```python
from build123d import *

# Parameters (mm, degrees)
SKETCH1_W                                    = 110
SKETCH1_H                                    = 30
EXTRUDE1_DEPTH                               = 2
CUT_EXTRUDE1_DEPTH                           = 3
CHAMFER1_SIZE                                = 9
CHAMFER1_SIZE2                               = 1.5
CSK_FOR_M3_COUNTERSUNK_RAISED_HEAD_S_2_COUNT = 2
CSK_FOR_M3_COUNTERSUNK_RAISED_HEAD_S_2_PITCH = 95
CSK_FOR_M3_COUNTERSUNK_RAISED_HEAD_S_3_COUNT = 2
CSK_FOR_M3_COUNTERSUNK_RAISED_HEAD_S_3_PITCH = 97.082439195
CSK_FOR_M3_COUNTERSUNK_RAISED_HEAD_S_4_COUNT = 2
CSK_FOR_M3_COUNTERSUNK_RAISED_HEAD_S_4_PITCH = 20
M3_TAPPED_HOLE1_D                            = 3


with BuildPart() as part:
    # Sketch1 → Extrude1 (new body)
    with BuildSketch(Plane(origin=(0, 0, 0), x_dir=(1, 0, 0), z_dir=(0, 1, 0))):
        Rectangle(SKETCH1_W, SKETCH1_H)
    extrude(amount=EXTRUDE1_DEPTH)

    # Sketch2 → Cut-Extrude1 (cut, through all)
    with BuildSketch(Plane(origin=(0, 2, 0), x_dir=(-1, 0, 0), z_dir=(0, 1, 0))):
        with BuildLine():
            Line((5, 0), (5, -15))
            Line((5, -15), (-5, -15))
            Line((-5, -15), (-5, 0))
            ThreePointArc((-5, 0), (0, 5), (5, 0))
        make_face()
    extrude(amount=-CUT_EXTRUDE1_DEPTH, mode=Mode.SUBTRACT)

    # Chamfer1
    chamfer1_edges = [part.edges().sort_by_distance(p)[0] for p in [
        (0, 2, 5),
        (5, 2, -7.5),
        (-5, 2, -7.5),
    ]]
    chamfer1_side = [part.faces().sort_by_distance(p)[0] for p in [
        (-53.859824575, 2, 0),
    ]]
    chamfer(chamfer1_edges, length=CHAMFER1_SIZE, length2=CHAMFER1_SIZE2, reference=chamfer1_side[0])

    # Sketch8 → CSK for M3 Countersunk Raised Head Screw1 (revolve, cut)
    with BuildSketch(Plane(origin=(47.5, 0, -10), x_dir=(0, 0, -1), z_dir=(1, 0, 0))):
        Polygon((0, 0), (0, 2), (1.7, 2), (1.7, 1.45), (3.15, 0), align=None)
    csk_for_m3_countersunk_raised_head_screw = revolve(axis=Axis((47.5, -6.35, -10), (0, 1, 0)), mode=Mode.SUBTRACT)

    # CSK for M3 Countersunk Raised Head S 2: CSK for M3 Countersunk Raised Head Screw1 ×2
    with Locations(*[(-i * CSK_FOR_M3_COUNTERSUNK_RAISED_HEAD_S_2_PITCH, 0, 0) for i in range(1, CSK_FOR_M3_COUNTERSUNK_RAISED_HEAD_S_2_COUNT)]):
        add(csk_for_m3_countersunk_raised_head_screw, mode=Mode.SUBTRACT)

    # CSK for M3 Countersunk Raised Head S 3: CSK for M3 Countersunk Raised Head Screw1 ×2
    with Locations(*[Vector(-0.978549785, 0, 0.206010481) * (i * CSK_FOR_M3_COUNTERSUNK_RAISED_HEAD_S_3_PITCH) for i in range(1, CSK_FOR_M3_COUNTERSUNK_RAISED_HEAD_S_3_COUNT)]):
        add(csk_for_m3_countersunk_raised_head_screw, mode=Mode.SUBTRACT)

    # CSK for M3 Countersunk Raised Head S 4: CSK for M3 Countersunk Raised Head Screw1 ×2
    with Locations(*[(0, 0, i * CSK_FOR_M3_COUNTERSUNK_RAISED_HEAD_S_4_PITCH) for i in range(1, CSK_FOR_M3_COUNTERSUNK_RAISED_HEAD_S_4_COUNT)]):
        add(csk_for_m3_countersunk_raised_head_screw, mode=Mode.SUBTRACT)

    # M3 Tapped Hole1 (through all)
    with Locations(Plane(origin=(0, 2, 0), x_dir=(-1, 0, 0), z_dir=(0, 1, 0))):
        with Locations((-30, 0), (30, 0)):
            Hole(M3_TAPPED_HOLE1_D / 2)


solid = part.part
```
Geometry check sheet. Reference: the model listing, model coordinates, mm. A direction names the side the tool comes from. Round coordinates to 2 decimals unless told otherwise and drop trailing zeros. Order: outer loops, then holes, each group sorted by start corner. A loop starts at its lowest first (then second) coordinate and runs counter-clockwise, first axis right, second up. Notation, with made-up numbers: (43.5, 76) - (71.5, 76) arc R27 ccw to (71.5, 104) - close; hole circle Ø6 at (75.5, 65). An arc over 180 degrees is marked (long way). Use a Markdown table: item, result. Add a question column.
1) Section check A-A (x = -47.5). Record the cut outline in (y, z), then the cut area to 3 significant figures.
2) Mould release check, pull along Z, two halves, no side actions. Record for faces 1 (the flat face through (-13, 2, 6)), 2 (the cylindrical face through (49.16, 1.72, -9.63)), 3 (the cylindrical face through (0.1, 0.3, 5)), 4 (the cylindrical face through (-49.186, 1.721, 10.221)): released by +Z, released by -Z, zero draft, split by the parting line, or undercut.
3) Thickness scan on line 1 along Z through (x, y) = (-47.5, 1.8); line 2 along Z through (x, y) = (-30, 1.4); line 3 along Y through (x, z) = (9, 5.5). Record the ranges inside material, lowest first.
4) Section check C-C (x = -30). Record the cut outline in (y, z), then the cut area to 3 significant figures.
5) Gauge pin test, flat ends, axial feed: P1, Ø4, axis at x = -30, z = 0, coming from the +Y side; P2, Ø4, axis at x = 47.5, z = 10, coming from the -Y side; P3, Ø12, axis at x = 4, z = -5, coming from the +Y side. Record the tip position at first contact, or that the pin passes through.
6) Section check B-B (z = -4.5). Record the cut outline in (x, y).
7) Set-up check for faces 5 (the cylindrical face through (-45.84, 1.72, -9.63)), 6 (the flat face through (-9.44, 1.24, -7.4)): record each of +Z, -Z, +X, -X, +Y, -Y from which the full face is reachable in a straight line by a thin tool's end or side.
8) Section check D-D (z = -10). Record the cut outline in (x, y), then the cut area to 3 significant figures.
Established:
| question | item | result |
|---|---|---|
| 1 | outline | (0, -15) - (2, -15) - (2, -11.7) - (1.45, -11.7) - (0, -13.15) - close; (0, -6.85) - (1.45, -8.3) - (2, -8.3) - (2, 8.3) - (1.45, 8.3) - (0, 6.85) - close; (0, 13.15) - (1.45, 11.7) - (2, 11.7) - (2, 15) - (0, 15) - close |
| 1 | area | 42.2 mm2 |
| 2 | face 1 | zero draft |
| 2 | face 2 | undercut |
| 2 | face 3 | released by -Z |
| 2 | face 4 | undercut |
| 3 | line 1 | -15 to -11.7, -8.3 to 8.3, 11.7 to 15 |
| 3 | line 2 | -15 to -1.5, 1.5 to 15 |
| 3 | line 3 | 0 to 1.42 |
| 4 | outline | (0, -15) - (2, -15) - (2, -1.5) - (0, -1.5) - close; (0, 1.5) - (2, 1.5) - (2, 15) - (0, 15) - close |
| 4 | area | 54.0 mm2 |
| 5 | P1 | y = 2 |
| 5 | P2 | y = 1.15 |
| 5 | P3 | y = 1.33 |
| 6 | outline | (-55, 0) - (-5, 0) - (-5, 0.5) - (-14, 2) - (-55, 2) - close; (5, 0) - (55, 0) - (55, 2) - (14, 2) - (5, 0.5) - close |
| 7 | face 5 | +Y, -Y |
| 7 | face 6 | -Z, +Y |
| 8 | outline | (-55, 0) - (-50.65, 0) - (-49.2, 1.45) - (-49.2, 2) - (-55, 2) - close; (-45.8, 1.45) - (-44.35, 0) - (-5, 0) - (-5, 0.5) - (-14, 2) - (-45.8, 2) - close; (5, 0) - (44.35, 0) - (45.8, 1.45) - (45.8, 2) - (14, 2) - (5, 0.5) - close; (49.2, 1.45) - (50.65, 0) - (55, 0) - (55, 2) - (49.2, 2) - close |
| 8 | area | 169 mm2 |
